Study the drawing (mm; zero at the part's minimum x, y, z) and answer. A direction names the side the tool comes from. Give positions to 0.01 mm unless a question says otherwise; leave off trailing zeros. Order: outer loops, then holes, each group sorted by start corner. A loop starts at its lowest first (then second) coordinate and runs counter-clockwise, first axis right, second up.
Item 1: Which of the six approach directions +Z, -Z, +X, -X, +Y, -Y give full straight-line access (tool end or side, diameter ignored) to the marked faces 4, 5 and 6?
Item 2: A cutting plane is placed at D-D (x = 5). Write down the section's boundary in (y, z) (1 decimal).
Item 3: The mould has two halves that part along X. Classify the marked faces 1, 2 and 3: +X half, -X half, draft (parallel to the pull), parting line (faces both ways), or undercut.
Item 4: Given pin 1 Ø1.5 at (x, z) = (69, 8) entering from -Y; pin 2 Ø1 at (x, y) = (53, 7.5) entering from +Z; pin 3 Ø1 at (x, z) = (40, 4) entering from -Y, each flat-ended and moving along its own axis, determine where each tip first touches the part or whether it passes through.
Item 5: A cutting plane is placed at B-B (x = 18). Write down the section's boundary in (y, z), plus the area to 3 significant figures.
Item 6: Find the intervals of material crossed by line 1 along X through (y, z) = (2, 7.75) (1 decimal); line 2 along X through (y, z) = (4, 7.25); line 3 along X through (y, z) = (11.25, 12.75), in increasing order.
Item 7: A cutting plane is placed at A-A (y = 6). Write down the section's boundary in (x, z).
Item 8: A cutting plane is placed at C-C (y = 10). Write down the section's boundary in (x, z) (1 decimal).
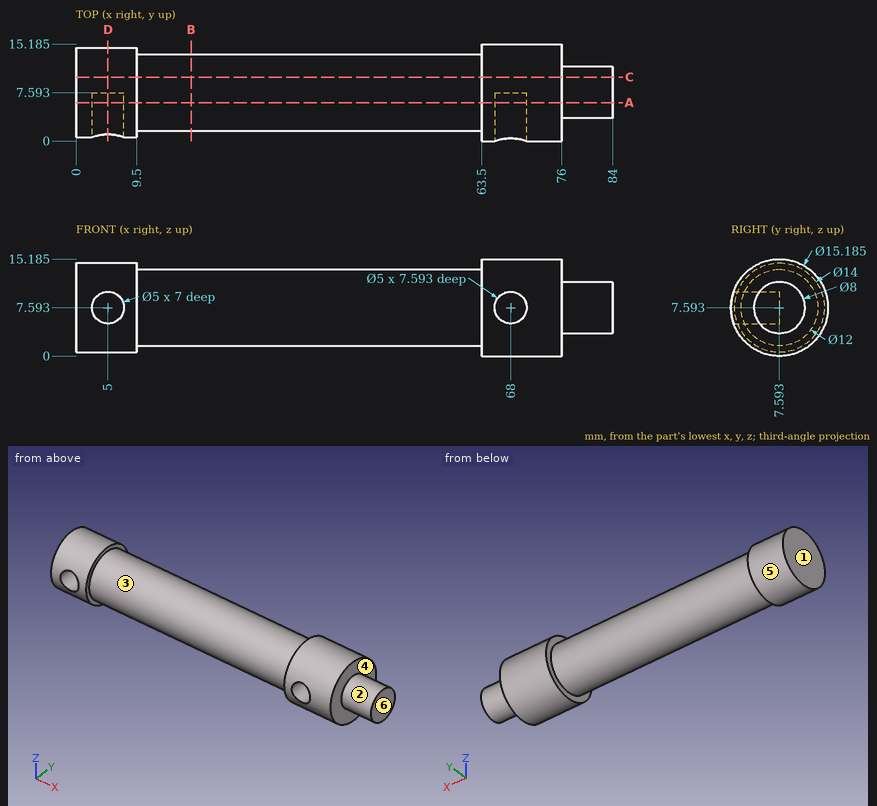
Response values:
1. face 4: +X
1. face 5: -X
1. face 6: +Z, -Z, +X, +Y, -Y
2. outline: (1.1, 5.1) arc R7 ccw (long way) to (1.1, 10.1) - (7.6, 10.1) - (7.6, 5.1) - close
3. face 1: -X half
3. face 2: draft
3. face 3: undercut
4. pin 1: stops at y = 7.59
4. pin 2: stops at z = 13.59
4. pin 3: stops at y = 2.45
5. outline: circle Ø12 at (7.59, 7.59)
5. area: 113 mm2
6. line 1: x = 0 to 2.5, 7.5 to 65.5, 70.5 to 76
6. line 2: x = 0 to 2.52, 7.48 to 65.52, 70.48 to 84
6. line 3: x = 0 to 9.5, 63.5 to 76
7. outline: (0, 0.78) - (9.5, 0.78) - (9.5, 1.81) - (63.5, 1.81) - (63.5, 0.17) - (76, 0.17) - (76, 3.92) - (84, 3.92) - (84, 11.26) - (76, 11.26) - (76, 15.02) - (63.5, 15.02) - (63.5, 13.38) - (9.5, 13.38) - (9.5, 14.41) - (0, 14.41) - close; hole circle Ø5 at (5, 7.59); hole circle Ø5 at (68, 7.59)
8. outline: (0, 1) - (9.5, 1) - (9.5, 2.1) - (63.5, 2.1) - (63.5, 0.4) - (76, 0.4) - (76, 4.4) - (84, 4.4) - (84, 10.8) - (76, 10.8) - (76, 14.8) - (63.5, 14.8) - (63.5, 13.1) - (9.5, 13.1) - (9.5, 14.2) - (0, 14.2) - close
